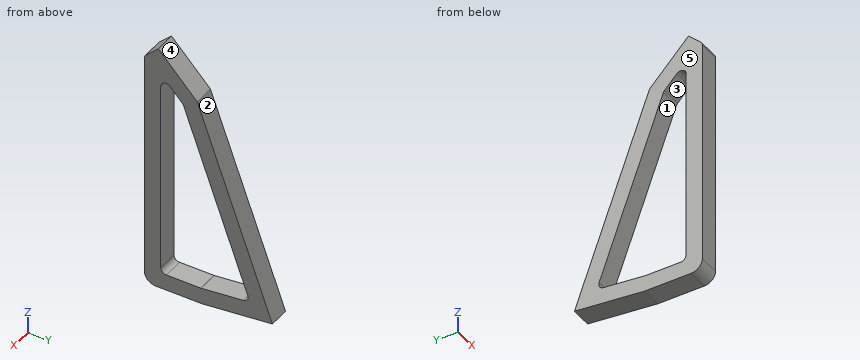
from build123d import *

# Parameters (mm, degrees)
BOSS_EXTRUDE1_DEPTH = 15


with BuildPart() as part:
    # Sketch1 → Boss-Extrude1 (new body)
    with BuildSketch(Plane(origin=(0, 0, 0), x_dir=(0, 0, -1), z_dir=(1, 0, 0))):
        with BuildLine():
            Line((-80.764356581, 24.012047683), (70.985255082, 79.244389389))
            Line((70.985255082, 79.244389389), (77.475739843, 27.555189639))
            Line((77.475739843, 27.555189639), (78.259876122, -6.675276303))
            ThreePointArc((78.259876122, -6.675276303), (75.98323725, -12.450192398), (70.261974321, -14.858488677))
            Line((70.261974321, -14.858488677), (-98.699643506, -14.858488677))
            ThreePointArc((-98.699643506, -14.858488677), (-100.257936009, -14.542470826), (-101.570004389, -13.644350914))
            Line((-101.570004389, -13.644350914), (-110.297725107, -4.651907634))
            Line((-110.297725107, -4.651907634), (-80.764356581, 24.012047683))
        make_face()
        with BuildLine():
            Line((-73.444540709, 13.906109511), (56.240883381, 61.107743698))
            ThreePointArc((56.240883381, 61.107743698), (59.694282591, 60.762394692), (61.577797623, 57.847329826))
            Line((61.577797623, 57.847329826), (65.468609196, 26.861518446))
            ThreePointArc((65.468609196, 26.861518446), (65.488687358, 26.660789803), (65.498619942, 26.45930416))
            Line((65.498619942, 26.45930416), (66.105012162, 1.237653648))
            ThreePointArc((66.105012162, 1.237653648), (64.968384485, -1.652717614), (62.106167747, -2.858488677))
            Line((62.106167747, -2.858488677), (-81.355445731, -2.858488677))
            ThreePointArc((-81.355445731, -2.858488677), (-85.062293687, -0.36157824), (-84.141307968, 4.011872206))
            Line((-84.141307968, 4.011872206), (-74.862322373, 13.017699911))
            ThreePointArc((-74.862322373, 13.017699911), (-74.200401783, 13.53686287), (-73.444540709, 13.906109511))
        make_face(mode=Mode.SUBTRACT)
    extrude(amount=BOSS_EXTRUDE1_DEPTH)


solid = part.part
Build history of the part. All positions in model axes, mm. Face numbers are marked on the shaded views. A direction names the side the tool comes from. Round coordinates to 2 decimals unless told otherwise and drop trailing zeros. Loops run counter-clockwise (first coordinate to the right, second up) from the corner with the lowest first, then second, coordinate; pieces in that order, holes last. Notation, with made-up numbers: (7.5, 41) -> (28.5, 41) arc R12 cw to (28.5, 52) -> close; hole circle Ø2 at (3, 15.25). An arc over 180 degrees is marked (long way). Answer in a Markdown table with one row per item.
Item 1: Which spindle directions (+Z, -Z, +X, -X, +Y, -Y) get a long thin tool onto all of the face, cutting with end or side? Do the marked faces 1 and 2. Say none if no direction does.
Answers below:
| item | result |
|---|---|
| face 1 | +X, -X |
| face 2 | +Z, +X, -X, +Y |
Item 2: Mould opens along Y. For the marked faces 3, 4 and 5 say: +Y half, -Y half, draft (parallel to the pull), parting line (faces both ways), or undercut.
Answers below:
| item | result |
|---|---|
| face 3 | undercut |
| face 4 | +Y half |
| face 5 | draft |
Item 3: Drill centre lines: L1, parallel to Y at x = 14.25, z = 85; L2, parallel to Y at x = 13.5, z = -2; L3, parallel to Z at x = 3.5, y = 12.5. Where is each one in solid material? Low to high. Write a range as [from, to].
Answers below:
| item | result |
|---|---|
| L1 | y = [-14.86, -0.51], [2.79, 19.9] |
| L2 | y = [-14.86, -2.86], [41.37, 54.14] |
| L3 | z = [-77.82, -65.83], [75.4, 92.63] |
Item 4: Pin check, flat tips, straight feed: pin 1 (1 mm diameter, centred on x = 7.5, z = -11.5, fed in from +Y); pin 2 (6 mm diameter, centred on x = 5, y = 12, fed in from +Z); pin 3 (1.5 mm diameter, centred on x = 11.5, z = 77, fed in from +Y). Stop position of each tip, or through.
Answers below:
| item | result |
|---|---|
| pin 1 | stops at y = 57.78 |
| pin 2 | stops at z = 96.23 |
| pin 3 | stops at y = 25.66 |
Item 5: Saw through at D-D (y = 64). Write the cut outline in (x, z).
Answers below:
| item | result |
|---|---|
| outline | (0, -72.9) -> (15, -72.9) -> (15, -29.1) -> (0, -29.1) -> close |
Item 6: Saw through at B-B (y = -1). Write the cut outline in (x, z), and give its area (3 significant figures).
Answers below:
| item | result |
|---|---|
| outline | (0, -78.13) -> (15, -78.13) -> (15, -65.48) -> (0, -65.48) -> close; (0, 84.73) -> (15, 84.73) -> (15, 106.54) -> (0, 106.54) -> close |
| area | 517 mm² |
Item 7: Saw through at A-A (x = 3). Write the cut outline in (y, z), and give its area (3 significant figures).
Answers below:
| item | result |
|---|---|
| outline | (-14.86, -70.26) arc R8 ccw to (-6.68, -78.26) -> (27.56, -77.48) -> (79.24, -70.99) -> (24.01, 80.76) -> (-4.65, 110.3) -> (-13.64, 101.57) arc R4 ccw to (-14.86, 98.7) -> close; hole (-2.86, -62.11) arc R4 ccw to (1.24, -66.11) -> (26.46, -65.5) arc R4 ccw to (26.86, -65.47) -> (57.85, -61.58) arc R4 ccw to (61.11, -56.24) -> (13.91, 73.44) arc R4 ccw to (13.02, 74.86) -> (4.01, 84.14) arc R4 ccw to (-2.86, 81.36) -> close |
| area | 5,320 mm² |
Item 8: Saw through at C-C (z = 77). Write the cut outline in (x, y).
Answers below:
| item | result |
|---|---|
| outline | (0, -14.86) -> (15, -14.86) -> (15, -2.86) -> (0, -2.86) -> close; (0, 10.94) -> (15, 10.94) -> (15, 25.38) -> (0, 25.38) -> close |
